```python
from build123d import *

# Parameters (mm, degrees)
CUT_EXTRUDE1_REACH = 29.279
CHAMFER1_SIZE      = 0.25
FILLET1_R          = 0.2


with BuildPart() as part:
    # Sketch1 → Revolve1 (revolve)
    with BuildSketch(Plane(origin=(0, 0, 0), x_dir=(0, 0, -1), z_dir=(1, 0, 0)), mode=Mode.PRIVATE) as revolve1_sk:
        Polygon((0, 1.5), (0, 2.75), (-2, 2.75), (-2, 0), (25, 0), (25, 1.5), align=None)
    revolve(revolve1_sk.sketch.rotate(Axis((0, 0, 13.782385085), (0, 0, -1)), 90), axis=Axis((0, 0, 13.782385085), (0, 0, -1)))

    # Sketch2 → Cut-Revolve1 (revolve, cut)
    with BuildSketch(Plane(origin=(0, 0, 0), x_dir=(0, 0, -1), z_dir=(1, 0, 0)), mode=Mode.PRIVATE) as cut_revolve1_sk:
        Polygon((0.077350269, 0), (-0.5, 1), (-2, 1), (-2, 0), align=None)
    revolve(cut_revolve1_sk.sketch.rotate(Axis((0, 0, 0), (0, 0, 1)), 90), axis=Axis((0, 0, 0), (0, 0, 1)), mode=Mode.SUBTRACT)

    # Cut-Extrude1: up to this cone (the profile starts inside it)
    cut_extrude1_end = Plane(origin=(0, 0, 2), z_dir=(0, 0, 1)).offset(-2.077349269) * Cone(1.732e-06, 61.408868018, 35.454425481, align=(Align.CENTER, Align.CENTER, Align.MIN), mode=Mode.PRIVATE)
    # Sketch3 → Cut-Extrude1 (cut, up to the surface)
    with BuildSketch(Plane.XY.offset(2), mode=Mode.PRIVATE) as cut_extrude1_sk1:
        Polygon((0, 1.154700538), (-1, 0.577350269), (-1, -0.577350269), (0, -1.154700538), (1, -0.577350269), (1, 0.577350269), align=None)
    cut_extrude1_tool1 = extrude(cut_extrude1_sk1.sketch, amount=-CUT_EXTRUDE1_REACH, mode=Mode.PRIVATE) & cut_extrude1_end
    add(cut_extrude1_tool1.solids().sort_by_distance((0, 0, 2))[0], mode=Mode.SUBTRACT)

    # Sketch4 → Cut-Revolve2 (revolve, cut)
    with BuildSketch(Plane(origin=(0, 0, 0), x_dir=(0, 0, -1), z_dir=(1, 0, 0)), mode=Mode.PRIVATE) as cut_revolve2_sk:
        Polygon((-1.5, 0.866025404), (-2.5, 0.866025404), (-2.5, 1.443375673), align=None)
    revolve(cut_revolve2_sk.sketch.rotate(Axis((0, 0, 0), (0, 0, 1)), 270), axis=Axis((0, 0, 0), (0, 0, 1)), mode=Mode.SUBTRACT)

    # Chamfer1
    chamfer1_edges = [part.edges().sort_by_distance(p)[0] for p in [
        (-1.5, 0, -25),
    ]]
    chamfer(chamfer1_edges, length=CHAMFER1_SIZE)

    # Fillet1
    fillet1_edges = [part.edges().sort_by_distance(p)[0] for p in [
        (-2.75, 0, 2),
    ]]
    fillet(fillet1_edges, radius=FILLET1_R)


solid = part.part
```
Verification items for the finished model (mm, model axes). A direction names the side the tool comes from. Round coordinates to 2 decimals unless told otherwise and drop trailing zeros. Write each loop counter-clockwise with the first axis right and the second up, starting at its lowest first coordinate (ties: lowest second). Pieces come first, ordered by that corner, then holes. Notation, with made-up numbers: (-36.75, 45) -> (-23.75, 45) arc R29 cw to (-23.75, 77) -> close; hole circle Ø3 at (64, -0.75). An arc over 180 degrees is marked (long way). Write each question's results on one line, items separated by ' | '. Start each with the question number.
1. Draft check along Y on faces 3 (the cylindrical face through (1.43, -0.45, -12.2)), 4 (the flat face through (-1.2, 1.2, 0)), 5 (the flat face through (-1, 0, 1)). Enter one of: +Y half, -Y half, draft (parallel to the pull), parting line (faces both ways), or undercut.
2. Cross-section at A-A (z = -21.25). Enter the section's corners in (x, y), then the cut area to 3 significant figures.
3. Set-up check for faces 1 (the flat face through (0, 0, -25)), 2 (the flat face through (1, 0, 1)): record each of +Z, -Z, +X, -X, +Y, -Y from which the full face is reachable in a straight line by a thin tool's end or side.
4. Material ranges on probe 1 along Y at (x, z) = (0.1, -0.75); probe 2 along Y at (x, z) = (-0.15, 1.25), recorded low to high. Write a range as from..to.
5. Depth check by flat-ended pin: P1, Ø0.6, axis at y = -0.5, z = 1.5, coming from the -X side; P2, Ø1.5, axis at y = 0, z = -4.5, coming from the -X side; P3, Ø2, axis at x = 2, z = -10.5, coming from the +Y side. Enter the tip coordinate at first touch or a pass-through.
Solutions:
1) face 3: parting line | face 4: draft | face 5: undercut
2) outline: circle Ø3 at (0, 0) | area: 7.07 mm2
3) face 1: -Z, +X, -X, +Y, -Y | face 2: +Z
4) probe 1: y = -1.5..1.5 | probe 2: y = -2.75..-1.07, 1.07..2.75
5) P1: stops at x = -2.74 | P2: stops at x = -1.5 | P3: stops at y = 1.12
